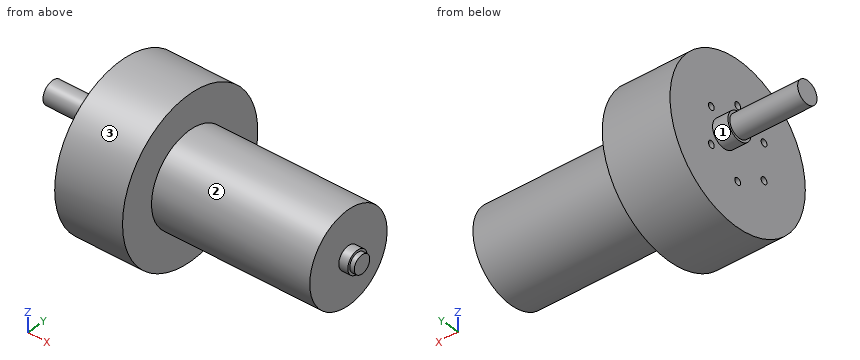
```python
from build123d import *

# Parameters (mm, degrees)
SKETCH2_R           = 6
BOSS_EXTRUDE1_DEPTH = 6.8
SKETCH3_R           = 5
BOSS_EXTRUDE2_DEPTH = 30
SKETCH4_R           = 1.5
CUT_EXTRUDE1_DEPTH  = 3


with BuildPart() as part:
    # Sketch1 → Revolve1 (revolve)
    with BuildSketch(Plane.XY, mode=Mode.PRIVATE) as revolve1_sk:
        Polygon((70.300682485, 4), (70.300682485, 5), (66.300682485, 5), (66.300682485, 20), (-3.699317515, 20), (-3.699317515, 35), (-33.699317515, 35), (-33.699317515, 0), (72.300682485, 0), (72.300682485, 4), align=None)
    revolve(revolve1_sk.sketch.rotate(Axis((-33.699317515, 0, 0), (1, 0, 0)), 180), axis=Axis((-33.699317515, 0, 0), (1, 0, 0)))

    # Sketch2 → Boss-Extrude1 (add)
    with BuildSketch(Plane.ZY.offset(33.699317515)):
        with Locations(Location((0, 7, 0), (0, 0, 90))):
            Circle(SKETCH2_R)
    extrude(amount=BOSS_EXTRUDE1_DEPTH)

    # Sketch3 → Boss-Extrude2 (add)
    with BuildSketch(Plane.ZY.offset(40.499317515)):
        with Locations((0, 7)):
            Circle(SKETCH3_R)
    extrude(amount=BOSS_EXTRUDE2_DEPTH)

    # Sketch4 → Cut-Extrude1 (cut)
    with BuildSketch(Plane.ZY.offset(33.699317515)):
        with Locations((-15.75, 0)):
            Circle(SKETCH4_R)
        with Locations((-7.875, 13.63990011)):
            Circle(SKETCH4_R)
        with Locations((7.875, 13.63990011)):
            Circle(SKETCH4_R)
        with Locations((15.75, 0)):
            Circle(SKETCH4_R)
        with Locations((7.875, -13.63990011)):
            Circle(SKETCH4_R)
        with Locations((-7.875, -13.63990011)):
            Circle(SKETCH4_R)
    extrude(amount=-CUT_EXTRUDE1_DEPTH, mode=Mode.SUBTRACT)


solid = part.part
```
The listing builds one solid part. Answer for the finished solid, in the listing's coordinates (mm). Face numbers are marked on the shaded views. A direction names the side the tool comes from. Give positions to 0.01 mm unless a question says otherwise; leave off trailing zeros. Order: outer loops, then holes, each group sorted by start corner. A loop starts at its lowest first (then second) coordinate and runs counter-clockwise, first axis right, second up. Notation, with made-up numbers: (23, 1) - (30, 1) arc R8 cw to (30, 6) - close; hole circle Ø3 at (-12, 40). An arc over 180 degrees is marked (long way). Answer in a Markdown table with one row per item. Add a question column.
Q1. Which of the six approach directions +Z, -Z, +X, -X, +Y, -Y give full straight-line access (tool end or side, diameter ignored) to the marked faces 1, 2 and 3?
Q2. The part is cut by section A-A (z = 0). Determine the outline of the cut face in (x, y).
Q3. The part is cut by section B-B (x = -43). Determine the outline of the cut face in (y, z).
Q4. The part is cut by section D-D (z = -15.75). Determine the outline of the cut face in (x, y).
Q5. Given P1, Ø4, axis at x = 52.5, z = -11, coming from the +Y side; P2, Ø21, axis at y = 0.5, z = 16.5, coming from the -X side; P3, Ø4, axis at y = 0, z = 15.75, coming from the +X side, each flat-ended and moving along its own axis, determine where each tip first touches the part or whether it passes through.
Q6. The part is cut by section C-C (y = -25). Determine the outline of the cut face in (x, z), then the cut area to 3 significant figures.
Q7. Find the intervals of material crossed by line 1 along Z through (x, y) = (18.5, -14); line 2 along X through (y, z) = (10.5, -30.5); line 3 along Z through (x, y) = (-22.5, 0.5), in increasing order. Write a range as [from, to].
Determined:
| question | item | result |
|---|---|---|
| 1 | face 1 | -X |
| 1 | face 2 | +X |
| 1 | face 3 | +X, -X |
| 2 | outline | (-70.5, 2) - (-40.5, 2) - (-40.5, 1) - (-33.7, 1) - (-33.7, -35) - (-3.7, -35) - (-3.7, -20) - (66.3, -20) - (66.3, -5) - (70.3, -5) - (70.3, -4) - (72.3, -4) - (72.3, 4) - (70.3, 4) - (70.3, 5) - (66.3, 5) - (66.3, 20) - (-3.7, 20) - (-3.7, 35) - (-33.7, 35) - (-33.7, 13) - (-40.5, 13) - (-40.5, 12) - (-70.5, 12) - close |
| 3 | outline | circle Ø10 at (7, 0) |
| 4 | outline | (-33.7, -31.26) - (-3.7, -31.26) - (-3.7, -12.33) - (66.3, -12.33) - (66.3, 12.33) - (-3.7, 12.33) - (-3.7, 31.26) - (-33.7, 31.26) - (-33.7, 1.5) - (-30.7, 1.5) - (-30.7, -1.5) - (-33.7, -1.5) - close |
| 5 | P1 | stops at y = 17.86 |
| 5 | P2 | stops at x = -33.7 |
| 5 | P3 | stops at x = 66.3 |
| 6 | outline | (-33.7, -24.49) - (-3.7, -24.49) - (-3.7, 24.49) - (-33.7, 24.49) - close |
| 6 | area | 1,470 mm² |
| 7 | line 1 | z = [-14.28, 14.28] |
| 7 | line 2 | x = [-33.7, -3.7] |
| 7 | line 3 | z = [-35, 35] |
